Autodesk Inventor part; units mm, degrees
ref_plane "YZ Plane" through (0, 0, 0) normal (1, 0, 0) x (0, 1, 0)
ref_plane "XZ Plane" through (0, 0, 0) normal (0, 1, 0) x (-1, 0, 0)
ref_plane "XY Plane" through (0, 0, 0) normal (0, 0, 1) x (1, 0, 0)
sketch "Sketch4" plane through (0, 0, 0) normal (0, 0, 1) x (1, 0, 0)
  circle A0 centre (0, 0) radius 505
  line L0 (0, 0) -> (0, 505)
  line L1 (0, 505) -> (0, 500)
  line L2 (0, 500) -> (25, 500)
  line L3 (0, 500) -> (-25, 500)
  line L4 (-25, 500) -> (-25, 450)
  line L5 (25, 500) -> (25, 450)
  line L6 (25, 450) -> (50, 450)
  line L7 (50, 450) -> (50, 502.5187)
  line L8 (-25, 450) -> (-50, 450)
  line L9 (-50, 450) -> (-50, 502.5187)
  line L10 (505, 0) -> (-505, 0)
  line L11 (-505, 0) -> (505, 0)
  line L12 (505, 0) -> (505, 62.2415)
  line L13 (505, 62.2415) -> (-505, 62.2415)
  line L14 (-505, 62.2415) -> (-505, 0)
  point P0 (-501.1497, 62.2415)
  point P1 (501.1497, 62.2415)
  dimension "d17" = 1010
  dimension "d18" = 5
  dimension "d19" = 25
  dimension "d20" = 25
  dimension "d22" = 50
  dimension "d23" = 50
  dimension "d24" = 25
  dimension "d25" = 25
  dimension "d36" = 62.2415
extrude "Extrusion4" add sketch "Sketch4" along normal blind 25 contours A0 L13 L0 L2 L5 L6 L7 | L9 L8 L4 L3 L0 L13 A0
sketch "Sketch5" plane through (25, 450, 0) normal (1, 0, 0) x (0, 0, -1)
  line L0 (-25, 0) -> (-25, 50)
  line L1 (-25, 50) -> (-12.5, 50) construction
  line L2 (0, 50) -> (-25, 50)
  line L3 (-12.5, 50) -> (-12.5, 37.5) construction
  circle A0 centre (-12.5, 37.5) radius 7.9375
  point P0 (0, -450)
  dimension "d28" = 12.5
  dimension "d29" = 15.875
extrude "Extrusion5" cut sketch "Sketch5" against normal up to surface (50 mm away)
sketch "Sketch6" plane through (-50, 450, 0) normal (0, 1, 0) x (1, 0, 0)
  line L0 (-455, -25) -> (555, -25)
  line L1 (0, 0) -> (0, -25)
  line L2 (25, -25) -> (0, -25)
  line L3 (0, -25) -> (0, 0)
  line L4 (0, 0) -> (25, 0)
  line L5 (25, 0) -> (25, -25)
  line L6 (75, 0) -> (100, 0)
  line L7 (100, 0) -> (100, -25)
  line L8 (100, -25) -> (75, -25)
  line L9 (75, -25) -> (75, 0)
  point P0 (50, 0)
extrude "Extrusion6" add sketch "Sketch6" along normal blind 25
extrude "Extrusion8" add sketch "Sketch4" along normal blind 12.5 contours A0 L10 L0 L13 | L0 L10 A0 L13
properties part number "Flap"
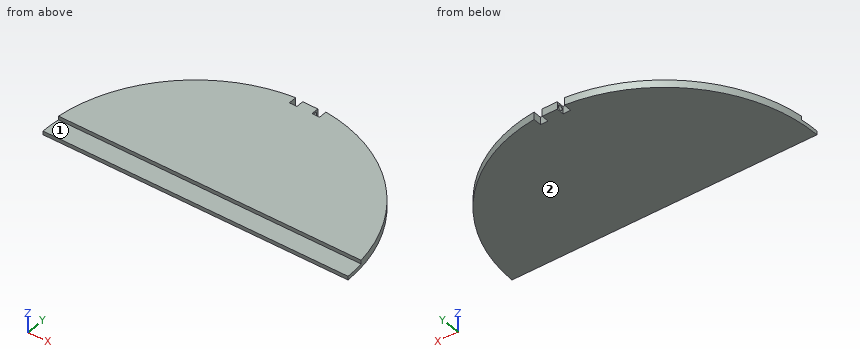
Geometry: final body of the model. Coordinates: model frame, mm. Face numbers are marked on the shaded views. A direction names the side the tool comes from. Coordinates: 2 decimals unless noted, no trailing zeros. Order: outer loops, then holes, each group sorted by start corner. A loop starts at its lowest first (then second) coordinate and runs counter-clockwise, first axis right, second up. Notation, with made-up numbers: M 21,51 L 54,51 A13 ccw 54,74 Z; hole C 3,18.25 d8. An arc over 180 degrees is marked long. One line per question, with ' | ' between items. Start each with the question number.
Item 1: Ray query, probe 1 along Z at (x, y) = (-99.5, 39); probe 2 along Y at (x, z) = (15.5, 6.5); probe 3 along Y at (x, z) = (-63.5, 21.5). Return the intervals inside material, ascending. Write a range as [from, to].
Item 2: Cut plane D-D, the plane x = 181. Return the cut outline in (y, z), then the cut area to 3 significant figures.
Item 3: Cut plane C-C, the plane y = 199. Return the cut outline in (x, z).
Item 4: Set-up query: the marked faces 1 and 2. Return all of +Z, -Z, +X, -X, +Y, -Y with unobstructed straight access to the full face (end or side cutting, diameter ignored); none if empty.
Item 5: Cut plane A-A, the plane x = -15. Return the cut outline in (y, z) (1 decimal).
Item 6: Pin query (flat end, axial travel): pin 1 Ø4 at (y, z) = (351, 12) entering from +X; pin 2 Ø2 at (y, z) = (105, 15.5) entering from +X; pin 3 Ø2 at (y, z) = (323.5, 11.5) entering from +X. Return the tip coordinate at first contact, or that it passes through.
Item 7: Cut plane B-B, the plane x = -232.5. Return the cut outline in (y, z).
A:
1) probe 1: z = [0, 12.5] | probe 2: y = [0, 482.3], [492.7, 500] | probe 3: y = [62.24, 500.99]
2) outline: M 0,0 L 471.45,0 L 471.45,25 L 62.24,25 L 62.24,12.5 L 0,12.5 Z | area: 11,000 mm2
3) outline: M -464.14,0 L 464.14,0 L 464.14,25 L -464.14,25 Z
4) face 1: +Z, +X, -X, -Y | face 2: -Z, +X, -X, +Y, -Y
5) outline: M 0,0 L 500,0 L 500,25 L 62.2,25 L 62.2,12.5 L 0,12.5 Z; hole C 487.5,12.5 d15.9
6) pin 1: stops at x = 365 | pin 2: stops at x = 494.18 | pin 3: stops at x = 388.61
7) outline: M 0,0 L 448.3,0 L 448.3,25 L 62.24,25 L 62.24,12.5 L 0,12.5 Z
